from build123d import *

# Parameters (mm, degrees)
SKETCH1_R           = 1
BOSS_EXTRUDE1_DEPTH = 4.5
REVOLVE1_ANGLE      = 180


with BuildPart() as part:
    # Sketch1 → Boss-Extrude1 (new, symmetric)
    with BuildSketch(Plane(origin=(0, 0, 0), x_dir=(1, 0, 0), z_dir=(0, 1, 0))):
        with Locations(Location((0, 0, 0), (0, 0, 270))):
            Circle(SKETCH1_R)
    extrude(amount=BOSS_EXTRUDE1_DEPTH, both=True)

    # Sketch2 → Revolve1 (revolve)
    with BuildSketch(Plane(origin=(0, 4.5, 0), x_dir=(1, 0, 0), z_dir=(0, 1, 0))):
        with BuildLine():
            Line((0, 1.2), (0, -1.2))
            ThreePointArc((0, -1.2), (-1.2, 0), (0, 1.2))
        make_face()
    revolve1 = revolve(axis=Axis((0, 4.5, -1.2), (0, 0, -1)), revolution_arc=REVOLVE1_ANGLE)

    # Mirror1: Revolve1 across plane
    add(revolve1.mirror(Plane.ZX))


solid = part.part
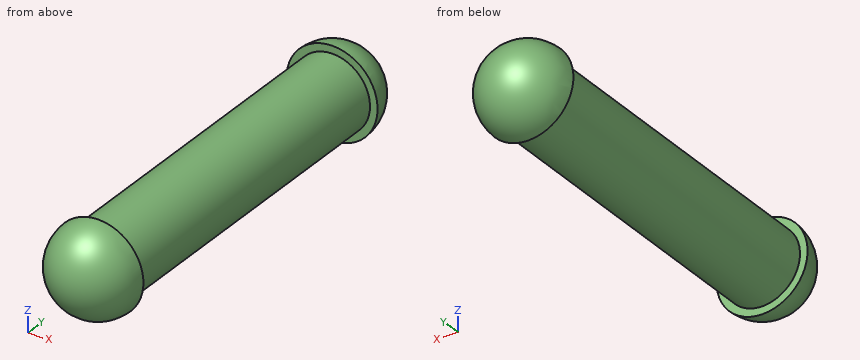
Read the model definition and answer for the solid it produces. Units are mm, in the model's axes. Coordinates: 2 decimals unless noted, no trailing zeros. Loops run counter-clockwise (first coordinate to the right, second up) from the corner with the lowest first, then second, coordinate; pieces in that order, holes last.
Q1. Consider probe 1 along X at (y, z) = (-2.5, -0.05); probe 2 along Y at (x, z) = (-0.1, 0.2); probe 3 along Y at (x, z) = (-0.35, -0.9). Determine where each line is inside the solid, lowest interval first.
Q2. The part is cut by section B-B on x = 0. Write down the section's boundary in (y, z).
Q3. The part is cut by section C-C on y = 2.25. Write down the section's boundary in (x, z).
Q4. The part is cut by section A-A on z = 0. Write down the section's boundary in (x, y).
Q5. This flat-tipped pin is pushed along its axis until it touches: pin 1 Ø1 at (x, y) = (-0.5, -3.5) entering from -Z. Where does it stop, or does it pass through?
Results below:
1. probe 1: x = -1 to 1
1. probe 2: y = -5.68 to 5.68
1. probe 3: y = -5.21 to 5.21
2. outline: (-4.5, -1.2) - (-4.5, -1) - (4.5, -1) - (4.5, -1.2) arc R1.2 ccw to (4.5, 1.2) - (4.5, 1) - (-4.5, 1) - (-4.5, 1.2) arc R1.2 ccw to start
3. outline: circle Ø2 at (0, 0)
4. outline: (-1.2, -4.5) arc R1.2 ccw to (1.2, -4.5) - (1, -4.5) - (1, 4.5) - (1.2, 4.5) arc R1.2 ccw to (-1.2, 4.5) - (-1, 4.5) - (-1, -4.5) - close
5. pin 1: stops at z = -1
